```python
from build123d import *

# Parameters (mm, degrees)
F0_R     = 3.175
F1_DEPTH = 19.05
F2_W     = 38.1
F2_H     = 19.05
F3_DEPTH = 6.35
F4_W     = 12.7
F4_H     = 19.05
F5_DEPTH = 6.35


with BuildPart() as f1:
    # F0 (on Top) → F1 (new body)
    with BuildSketch(Plane.XY):
        with BuildLine():
            Line((0, 50.8), (0, 0))
            Line((0, 0), (0, -12.7))
            Line((0, -12.7), (-133.35, -12.7))
            Line((-133.35, -12.7), (-133.35, -50.8))
            ThreePointArc((-133.35, -50.8), (-117.475, -34.925), (-101.6, -50.8))
            Line((-101.6, -50.8), (-101.6, -38.1))
            Line((-101.6, -38.1), (25.4, -38.1))
            Line((25.4, -38.1), (25.4, 0))
            Line((25.4, 0), (25.4, 25.4))
            Line((25.4, 25.4), (254, 25.4))
            Line((254, 25.4), (254, 50.8))
            Line((254, 50.8), (0, 50.8))
        make_face()
        with Locations((12.7, 6.35)):
            Circle(F0_R, mode=Mode.SUBTRACT)
    extrude(amount=F1_DEPTH)

    # F2 (on face) → F3 (join)
    with BuildSketch(Plane(origin=(-133.35, 0, 0), x_dir=(0, -1, 0), z_dir=(-1, 0, 0))):
        with Locations((31.75, 9.525)):
            Rectangle(F2_W, F2_H)
    extrude(amount=F3_DEPTH)

    # F4 (on face) → F5 (join)
    with BuildSketch(Plane.YZ.offset(-101.6)):
        with Locations((-44.45, 9.525)):
            Rectangle(F4_W, F4_H)
    extrude(amount=F5_DEPTH)


solid = f1.part
```
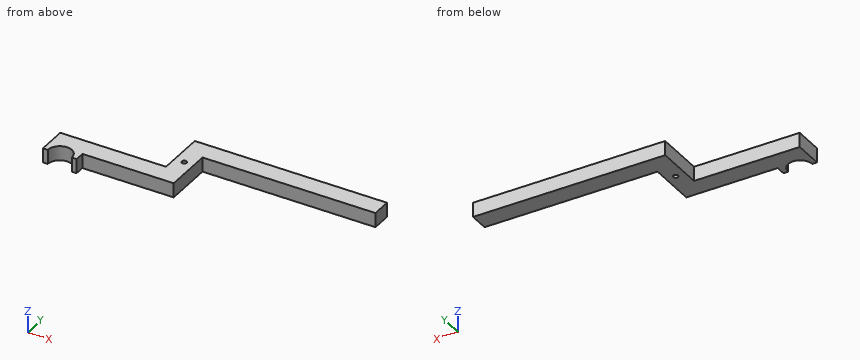
The listing builds one solid part. Answer for the finished solid, in the listing's coordinates (mm). Give positions to 0.01 mm unless a question says otherwise; leave off trailing zeros. Loops run counter-clockwise (first coordinate to the right, second up) from the corner with the lowest first, then second, coordinate; pieces in that order, holes last. Notation, with made-up numbers: M 10,-13.75 L 28,-13.75 A20 cw 28,0.25 Z; hole C -24,77 d2. An arc over 180 degrees is marked long. One line per item, written item: value.
Q1. Flat-ended cylindrical pins translate along their axes: P1, Ø6.5, axis at y = -46.5, z = 8, coming from the +X side; P2, Ø9.5, axis at x = 184.5, z = 5, coming from the -Y side; P3, Ø5.5, axis at y = 8.5, z = 12.5, coming from the +X side; P4, Ø5, axis at x = 117, y = 28.5, coming from the -Z side. Find the tip coordinate at first contact, or state that the pin passes through.
Working result:
P1: stops at x = -95.25
P2: stops at y = 25.4
P3: stops at x = 25.4
P4: stops at z = 0
Q2. A cutting plane is placed at B-B on x = 115. Determine the outline of the cut face in (y, z), then the cut area to 3 significant figures.
Working result:
outline: M 25.4,0 L 50.8,0 L 50.8,19.05 L 25.4,19.05 Z
area: 484 mm^2
Q3. A cutting plane is placed at C-C on y = 41. Determine the outline of the cut face in (x, z).
Working result:
outline: M 0,0 L 254,0 L 254,19.05 L 0,19.05 Z
Q4. Find the intervals of material crossed by line 1 (Y direction, x = 12.7, z = 6) (3 decimals); line 2 (X direction, y = -27, z = 14); line 3 (Y direction, x = 6.5, z = 13.75), in increasing order. Write a range as from..to.
Working result:
line 1: y = -38.1..3.175, 9.525..50.8
line 2: x = -139.7..25.4
line 3: y = -38.1..50.8
Q5. A cutting plane is placed at A-A on z = 13.5. Determine the outline of the cut face in (x, y) (3 decimals), then the cut area to 3 significant figures.
Working result:
outline: M -139.7,-50.8 L -133.35,-50.8 A15.875 cw -101.6,-50.8 L -95.25,-50.8 L -95.25,-38.1 L 25.4,-38.1 L 25.4,25.4 L 254,25.4 L 254,50.8 L 0,50.8 L 0,-12.7 L -139.7,-12.7 Z; hole C 12.7,6.35 d6.35
area: 11,700 mm^2
